Geometry check sheet. Reference: the model listing, model coordinates, mm. A direction names the side the tool comes from. Round coordinates to 2 decimals unless told otherwise and drop trailing zeros. Loops run counter-clockwise (first coordinate to the right, second up) from the corner with the lowest first, then second, coordinate; pieces in that order, holes last.
```python
from build123d import *

# Parameters (mm, degrees)
EXTRUDE_1_DEPTH             = 34.63
SKETCH_2_R                  = 2.6
CUT_EXTRUDE_1_DEPTH         = 106.56315361
EXTRUDE_2_DEPTH             = 3
SKETCH_4_W                  = 46.659566201
SKETCH_4_H                  = 12
SKETCH_4_R                  = 2.6
EXTRUDE_3_DEPTH             = 12.8
DRAFT_1_ANGLE               = 20
CUT_EXTRUDE_2_DEPTH         = 90.021233563
SKETCH_6_R                  = 3.6
CUT_EXTRUDE_3_DEPTH         = 28
FILLET_1_R                  = 5
CHAMFER_1_SIZE              = 5
DRAFT_1_OF_MIRROR_3_2_ANGLE = 20
CHAMFER_2_SIZE              = 5
FILLET_2_R                  = 5
SKETCH_7_W                  = 87.99
SKETCH_7_H                  = 3
EXTRUDE_4_DEPTH             = 12
SKETCH_8_R                  = 3.95
EXTRUDE_5_DEPTH             = 5
CHAMFER_3_SIZE              = 8
CHAMFER_4_SIZE              = 10
SKETCH_9_W                  = 19.5
SKETCH_9_H                  = 40
EXTRUDE_6_DEPTH             = 5
SKETCH_9_3_W                = 19.5
SKETCH_9_3_H                = 40
CUT_EXTRUDE_4_DEPTH         = 30
EXTRUDE_7_DEPTH             = 5
CHAMFER_5_SIZE              = 20
SKETCH_11_R                 = 1.25
CUT_EXTRUDE_5_DEPTH         = 5
SKETCH_12_R                 = 2.25
CUT_EXTRUDE_6_DEPTH         = 105.59373607


with BuildPart() as part:
    # Эскиз1 → Бобышка-Вытянуть1 (new body)
    with BuildSketch(Plane.XY):
        Polygon((-43.995, 3), (43.995, 3), (43.995, 33.32), (46.995, 33.32), (46.995, 0), (-46.995, 0), (-46.995, 33.32), (-43.995, 33.32), align=None)
    extrude(amount=EXTRUDE_1_DEPTH)

    # Эскиз2 → Вырез-Вытянуть1 (cut, through all)
    with BuildSketch(Plane.ZY.offset(46.995)):
        with Locations(Location((12.418647532, 22.211352468, 0), (0, 0, 270))):
            Circle(SKETCH_2_R)
        with Locations(Location((23.521352468, 22.211352468, 0), (0, 0, 270))):
            Circle(SKETCH_2_R)
        with Locations(Location((23.521352468, 11.108647532, 0), (0, 0, 270))):
            Circle(SKETCH_2_R)
    extrude(amount=-CUT_EXTRUDE_1_DEPTH, mode=Mode.SUBTRACT)

    # Эскиз3 → Бобышка-Вытянуть2 (add)
    with BuildSketch(Plane(origin=(0, 0, 0), x_dir=(1, 0, 0), z_dir=(0, 1, 0))):
        Polygon((-27.5, -34.63), (27.5, -34.63), (19.5, -69.26), (14.7, -69.26), (14.7, -40.26), (-14.7, -40.26), (-14.7, -69.26), (-19.5, -69.26), align=None)
    extrude(amount=EXTRUDE_2_DEPTH)

    # Эскиз4 → Бобышка-Вытянуть3 (add)
    with BuildSketch(Plane.ZY.offset(-14.7)):
        with Locations((45.9302169, 9)):
            Rectangle(SKETCH_4_W, SKETCH_4_H)
        with Locations((62.01, 9)):
            Circle(SKETCH_4_R, mode=Mode.SUBTRACT)
    extrude_3 = extrude(amount=-EXTRUDE_3_DEPTH)

    # Уклон1
    draft_1_faces = [part.faces().sort_by_distance(p)[0] for p in [
        (21.1, 9, 22.600433799),
    ]]
    draft(draft_1_faces, Plane(origin=(27.5, 15, 22.600433799), x_dir=(0, 0, 1), z_dir=(0, 1, 0)), DRAFT_1_ANGLE)

    # Эскиз5 → Вырез-Вытянуть2 (cut, through all)
    with BuildSketch(Plane.XZ.offset(-3)):
        Polygon((27.5, 34.63), (27.5, 69.26), (19.5, 69.26), align=None)
    cut_extrude_2 = extrude(amount=-CUT_EXTRUDE_2_DEPTH, mode=Mode.SUBTRACT)

    # Эскиз6 → Вырез-Вытянуть3 (cut)
    with BuildSketch(Plane(origin=(46.995, 0, 0), x_dir=(0, 0, -1), z_dir=(1, 0, 0))):
        with Locations(Location((-62.01, 9, 0), (0, 0, 90))):
            Circle(SKETCH_6_R)
    cut_extrude_3 = extrude(amount=-CUT_EXTRUDE_3_DEPTH, mode=Mode.SUBTRACT)

    # Скругление1
    fillet_1_edges = [part.edges().sort_by_distance(p)[0] for p in [
        (17.1, 15, 69.26),
    ]]
    fillet(fillet_1_edges, radius=FILLET_1_R)

    # Фаска1
    chamfer_1_edges = [part.edges().sort_by_distance(p)[0] for p in [
        (17.1, 0, 69.26),
    ]]
    chamfer(chamfer_1_edges, length=CHAMFER_1_SIZE)

    # Зеркальное отражение3: Бобышка-Вытянуть3, Вырез-Вытянуть2, Вырез-Вытянуть3 across plane
    add(extrude_3.mirror(Plane(origin=(0, 0, 0), x_dir=(0, 0, 1), z_dir=(1, 0, 0))))
    add(cut_extrude_2.mirror(Plane(origin=(0, 0, 0), x_dir=(0, 0, 1), z_dir=(1, 0, 0))), mode=Mode.SUBTRACT)
    add(cut_extrude_3.mirror(Plane(origin=(0, 0, 0), x_dir=(0, 0, 1), z_dir=(1, 0, 0))), mode=Mode.SUBTRACT)

    # Уклон1 of Mirror 3 2
    draft_1_of_mirror_3_2_faces = [part.faces().sort_by_distance(p)[0] for p in [
        (-21.1, 9, 22.600433799),
    ]]
    draft(draft_1_of_mirror_3_2_faces, Plane(origin=(-27.5, 15, 22.600433799), x_dir=(0, 0, 1), z_dir=(0, 1, 0)), DRAFT_1_OF_MIRROR_3_2_ANGLE)

    # Фаска2
    chamfer_2_edges = [part.edges().sort_by_distance(p)[0] for p in [
        (-17.1, 0, 69.26),
    ]]
    chamfer(chamfer_2_edges, length=CHAMFER_2_SIZE)

    # Скругление2
    fillet_2_edges = [part.edges().sort_by_distance(p)[0] for p in [
        (-17.1, 15, 69.26),
    ]]
    fillet(fillet_2_edges, radius=FILLET_2_R)

    # Эскиз7 → Бобышка-Вытянуть4 (add)
    with BuildSketch(Plane(origin=(0, 3, 0), x_dir=(1, 0, 0), z_dir=(0, 1, 0))):
        with Locations((0, -1.5)):
            Rectangle(SKETCH_7_W, SKETCH_7_H)
    extrude(amount=EXTRUDE_4_DEPTH)

    # Эскиз8 → Бобышка-Вытянуть5 (add)
    with BuildSketch(Plane.ZY.offset(-43.995)):
        Polygon((3, 3), (34.63, 3), (34.63, 33.32), (0, 33.32), (0, 15), (3, 15), align=None)
        with Locations((12.418647532, 22.211352468)):
            Circle(SKETCH_8_R, mode=Mode.SUBTRACT)
        with Locations((23.521352468, 22.211352468)):
            Circle(SKETCH_8_R, mode=Mode.SUBTRACT)
        with Locations((23.521352468, 11.108647532)):
            Circle(SKETCH_8_R, mode=Mode.SUBTRACT)
    extrude_5 = extrude(amount=EXTRUDE_5_DEPTH)

    # Зеркальное отражение4: Бобышка-Вытянуть5 across plane
    add(extrude_5.mirror(Plane(origin=(0, 0, 0), x_dir=(0, 0, 1), z_dir=(1, 0, 0))))

    # Фаска3
    chamfer_3_edges = [part.edges().sort_by_distance(p)[0] for p in [
        (42.995, 33.32, 34.63),
        (-42.995, 33.32, 34.63),
    ]]
    chamfer(chamfer_3_edges, length=CHAMFER_3_SIZE)

    # Фаска4
    chamfer_4_edges = [part.edges().sort_by_distance(p)[0] for p in [
        (38.995, 15, 1.5),
        (-38.995, 15, 1.5),
    ]]
    chamfer(chamfer_4_edges, length=CHAMFER_4_SIZE)

    # Эскиз9 → Бобышка-Вытянуть6 (add)
    with BuildSketch(Plane(origin=(6.8, 0, 0), x_dir=(0, 0, -1), z_dir=(1, 0, 0))):
        Polygon((-5, 3), (0, 3), (0, 10), (0, 50), (0, 57), (-5, 57), (-24.5, 57), (-29.5, 57), (-29.5, 50), (-29.5, 10), (-29.5, 3), (-24.5, 3), align=None)
        with Locations((-14.75, 30)):
            Rectangle(SKETCH_9_W, SKETCH_9_H, mode=Mode.SUBTRACT)
    extrude(amount=-EXTRUDE_6_DEPTH)

    # Эскиз9<3> → Вырез-Вытянуть4 (cut)
    with BuildSketch(Plane(origin=(6.8, 0, 0), x_dir=(0, 0, -1), z_dir=(1, 0, 0))):
        with Locations((-14.75, 30)):
            Rectangle(SKETCH_9_3_W, SKETCH_9_3_H)
    extrude(amount=CUT_EXTRUDE_4_DEPTH, mode=Mode.SUBTRACT)

    # Эскиз10 → Бобышка-Вытянуть7 (add)
    with BuildSketch(Plane(origin=(6.8, 0, 0), x_dir=(0, 0, -1), z_dir=(1, 0, 0))):
        Polygon((-29.5, 3), (-29.5, 57), (-40.26, 3), align=None)
    extrude(amount=-EXTRUDE_7_DEPTH)

    # Фаска5
    chamfer_5_edges = [part.edges().sort_by_distance(p)[0] for p in [
        (6.8, 15, 1.5),
        (1.8, 15, 1.5),
    ]]
    chamfer(chamfer_5_edges, length=CHAMFER_5_SIZE)

    # Эскиз11 → Вырез-Вытянуть5 (cut)
    with BuildSketch(Plane(origin=(6.8, 0, 0), x_dir=(0, 0, -1), z_dir=(1, 0, 0))):
        with Locations((-19.5, 54)):
            Circle(SKETCH_11_R)
        with Locations((-10, 54)):
            Circle(SKETCH_11_R)
    cut_extrude_5 = extrude(amount=-CUT_EXTRUDE_5_DEPTH, mode=Mode.SUBTRACT)

    # Зеркальное отражение5: Вырез-Вытянуть5 across plane
    add(cut_extrude_5.mirror(Plane.ZX.offset(30)), mode=Mode.SUBTRACT)

    # Эскиз12 → Вырез-Вытянуть6 (cut, through all)
    with BuildSketch(Plane(origin=(6.8, 0, 0), x_dir=(0, 0, -1), z_dir=(1, 0, 0))):
        with Locations(Location((-19.5, 6, 0), (0, 0, 180))):
            Circle(SKETCH_12_R)
        with Locations(Location((-10, 6, 0), (0, 0, 180))):
            Circle(SKETCH_12_R)
    extrude(amount=CUT_EXTRUDE_6_DEPTH, mode=Mode.SUBTRACT)


solid = part.part
```
1) Sectioned sample at A-A, the plane z = 55. Record the cut outline in (x, y).
Report:
outline: (-22.79, 0) - (-14.7, 0) - (-14.7, 15) - (-22.79, 15) - close; (14.7, 0) - (22.79, 0) - (22.79, 15) - (14.7, 15) - close
2) Sectioned sample at C-C, the plane x = 8. Record the cut outline in (y, z), then the cut area to 3 significant figures.
Report:
outline: (0, 0) - (33.8, 0) - (33.8, 3) - (3, 3) - (3, 40.26) - (0, 40.26) - close
area: 213 mm2
3) Mould release check, pull along X, two halves, no side actions. Record for faces 1 (the face through (18.995, 11, 64)), 2 (the face through (-1, 16, 0)), 3 (the face through (41.53, 26.128, 11.904)): +X half, -X half, draft (parallel to the pull), parting line (faces both ways), or undercut.
Report:
face 1: +X half
face 2: draft
face 3: undercut
4) Gauge pin test, flat ends, axial feed: pin 1 (16.5 mm diameter, centred on y = 6.5, z = 46, fed in from +X); pin 2 (6 mm diameter, centred on y = 8, z = 57, fed in from +X); pin 3 (8 mm diameter, centred on y = 8, z = 62.5, fed in from +X). Record the tip position at first contact, or that the pin passes through.
Report:
pin 1: stops at x = 26.78
pin 2: stops at x = 23.03
pin 3: stops at x = 21.99
5) Sectioned sample at D-D, the plane y = 46. Record the cut outline in (x, z), then the cut area to 3 significant figures.
Report:
outline: (1.8, 0) - (6.8, 0) - (6.8, 5) - (1.8, 5) - close; (1.8, 24.5) - (6.8, 24.5) - (6.8, 31.69) - (1.8, 31.69) - close
area: 61.0 mm2
6) Access from +Z, -Z, +X, -X, +Y, -Y to the whole of each face (thin tool, end or side, straight path). Record for faces 4 (the face through (-43.995, 8.5, 22.6)), 5 (the face through (-18.995, 11, 64)), 6 (the face through (-21.01, 8.916, 20.386)).
Report:
face 4: none
face 5: -X
face 6: +Y
7) Sectioned sample at B-B, the plane y = 54. Record the cut outline in (x, z).
Report:
outline: (1.8, 0) - (6.8, 0) - (6.8, 8.75) - (1.8, 8.75) - close; (1.8, 11.25) - (6.8, 11.25) - (6.8, 18.25) - (1.8, 18.25) - close; (1.8, 20.75) - (6.8, 20.75) - (6.8, 30.1) - (1.8, 30.1) - close
8) Scan lines: line 1 along Y through (x, z) = (2.8, 19.5); line 2 along Y through (x, z) = (20.3, 62.01); line 3 along X through (y, z) = (13, 14.5) (3 decimals). Record each from-to range of solid material in increasing order.
Report:
line 1: y = 0 to 4.75, 7.25 to 10, 50 to 52.75, 55.25 to 57
line 2: y = 0 to 5.4, 12.6 to 15
line 3: x = -46.995 to -38.995, 38.995 to 46.995
